```python
from build123d import *

# Parameters (mm, degrees)
SKETCH1_R            = 5.75
BOSS_EXTRUDE2_DEPTH  = 3
BOSS_EXTRUDE10_DEPTH = 0.15
CIRPATTERN1_COUNT    = 2
SKETCH5_R            = 2.5
CUT_EXTRUDE1_DEPTH   = 65.589571664
FILLET1_R            = 0.5
CHAMFER1_SIZE        = 1


with BuildPart() as part:
    # Sketch1 → Boss-Extrude2 (new, symmetric)
    with BuildSketch(Plane(origin=(0, 0, 0), x_dir=(1, 0, 0), z_dir=(0, 1, 0))):
        with Locations(Location((0, 0, 0), (0, 0, 270))):
            Circle(SKETCH1_R)
    extrude(amount=BOSS_EXTRUDE2_DEPTH, both=True)

    # Sketch4 → Boss-Extrude10 (add, symmetric)
    with BuildSketch(Plane(origin=(0, 0, 0), x_dir=(0.9743700647852351, -0.22495105434386553, 0), z_dir=(-0.22495105434386553, -0.9743700647852351, 0))):
        with BuildLine():
            Line((-10.409634183, 8.775037851), (-10.409634183, 60.5))
            ThreePointArc((-10.409634183, 60.5), (-9.530954526, 62.621320344), (-7.409634183, 63.5))
            Line((-7.409634183, 63.5), (-2.709478927, 63.5))
            ThreePointArc((-2.709478927, 63.5), (0.450679553, 62.374712683), (2.188403531, 59.505359351))
            add(Edge.make_bspline(
                [(4.983255085, 2.767158968), (7.368647348, 31.445436933), (2.188403531, 59.505359351)],
                knots=[0, 0, 0, 1, 1, 1], degree=2))
            ThreePointArc((4.983255085, 2.767158968), (0, 5.7), (-4.983255085, 2.767158968))
            Line((-4.983255085, 2.767158968), (-10.409634183, 8.775037851))
        make_face()
    boss_extrude10 = extrude(amount=BOSS_EXTRUDE10_DEPTH, both=True)

    # CirPattern1: Boss-Extrude10 ×2 about axis
    cirpattern1_axis = Axis((0, 3, 0), (0, -1, 0))
    for i in range(1, CIRPATTERN1_COUNT):
        add(boss_extrude10.rotate(cirpattern1_axis, i * 360 / CIRPATTERN1_COUNT))

    # Sketch5 → Cut-Extrude1 (cut, through all)
    with BuildSketch(Plane.XZ.offset(3)):
        with Locations(Location((0, 0, 0), (0, 0, 270))):
            Circle(SKETCH5_R)
    extrude(amount=-CUT_EXTRUDE1_DEPTH, mode=Mode.SUBTRACT)

    # Fillet1
    fillet1_edges = [part.edges().sort_by_distance(p)[0] for p in [
        (0, -3, -5.75),
        (0, 3, -5.75),
    ]]
    fillet(fillet1_edges, radius=FILLET1_R)

    # Chamfer1
    chamfer1_edges = [part.edges().sort_by_distance(p)[0] for p in [
        (0, 3, 2.5),
        (0, -3, 2.5),
    ]]
    chamfer(chamfer1_edges, length=CHAMFER1_SIZE)


solid = part.part
```
Here's how the part is built. I have some questions about the finished solid (model axes, mm). A direction names the side the tool comes from. Coordinates: 2 decimals unless noted, no trailing zeros. Order: outer loops, then holes, each group sorted by start corner. A loop starts at its lowest first (then second) coordinate and runs counter-clockwise, first axis right, second up.
1) Imagine slicing it at A-A on z = 0. List the corners of the cut face in (x, y) for me.
2) I need wall thicknesses on line 1 (X direction, y = 0.6, z = 0); line 2 (Y direction, x = -3.25, z = -33); line 3 (Y direction, x = -1.75, z = -5). Which ranges of each line are inside material? Lowest first, please.
3) Which directions (+Z, -Z, +X, -X, +Y, -Y) give clear straight access to the entire face, cutting with the end or side of a thin tool? Please do faces 1 (the face through (4, -3, 0)), 2 (the face through (-3.5, 0.04, -4.56)).
4) We'd pull the mould along X, two halves only. Please class faces 3 (the face through (-2.44, -0.03, 0.54)), 4 (the face through (4, 3, 0)): +X half, -X half, draft (parallel to the pull), parting line (faces both ways), or undercut.
5) Will this pin go through, and if not, where does the flat tip stop? pin 1 (1 mm diameter, centred on x = 3.5, z = 7.5, fed in from -Y).
Response values:
1. outline: (-5.75, -2.5) arc R0.5 ccw to (-5.25, -3) - (-3.5, -3) - (-2.5, -2) - (-2.5, 2) - (-3.5, 3) - (-5.25, 3) arc R0.5 ccw to (-5.75, 2.5) - close; (2.5, -2) - (3.5, -3) - (5.25, -3) arc R0.5 ccw to (5.75, -2.5) - (5.75, 2.5) arc R0.5 ccw to (5.25, 3) - (3.5, 3) - (2.5, 2) - close
2. line 1: x = -5.75 to -2.5, 2.5 to 5.75
2. line 2: y = -0.9 to -0.6
2. line 3: y = -3 to 3
3. face 1: +Z, -Z, +X, -X, -Y
3. face 2: none
4. face 3: undercut
4. face 4: draft
5. pin 1: stops at y = -1.08
